For this review, take the finished solid that the model builds, in its own axes (mm). A direction names the side the tool comes from. Coordinates: 2 decimals unless noted, no trailing zeros. Loops run counter-clockwise (first coordinate to the right, second up) from the corner with the lowest first, then second, coordinate; pieces in that order, holes last. Notation, with made-up numbers: (22.25, 54.5) - (39.25, 54.5) arc R22 ccw to (39.25, 62.5) - close; hole circle Ø5 at (-12.5, 53). An arc over 180 degrees is marked (long way). Answer as a JSON object with one key per item and string values. Group by question number.
Item 1: Mouldability with a two-part tool opening along Y and no side actions: class faces 4 (the cylindrical face through (49.3, -26.87, -24.56)), 5 (the flat face through (49, 60.038, 11)), 6 (the flat face through (110, -4, 9)), 7 (the cylindrical face through (-4.93, -0.03, 8.67)) as released by +Y, released by -Y, zero draft, split by the parting line, or undercut.
Item 2: Clearance check with flat-ended pins moving along their axes: pin 1 (1.5 mm diameter, centred on x = 58.5, z = 0, fed in from -Y); pin 2 (6 mm diameter, centred on x = 28, y = -36, fed in from +Z); pin 3 (3 mm diameter, centred on x = 46.5, y = -30, fed in from +Z). State where each tip first meets the part, or that it passes through.
Item 3: To check wall thickness, follow line 1 (Z direction, x = 20, y = 50); line 2 (Y direction, x = 33, z = 0.5); line 3 (Y direction, x = 51.5, z = 13.5). State the ranges of each line that lie inside material, in increasing order.
Item 4: We need section D-D (y = -14.5). Give the boundary of the cut face in (x, z), then the cut area to 3 significant figures.
Item 5: We need section A-A (z = -22). Give the boundary of the cut face in (x, y), then the cut area to 3 significant figures.
Item 6: We need section C-C (z = -8). Give the boundary of the cut face in (x, y).
Item 7: Tool access review of faces 1 (the flat face through (-10, -4, 9)), 2 (the cylindrical face through (104.93, -0.03, 8.67)), 3 (the flat face through (49, -7.459, -6)): name each direction out of +Z, -Z, +X, -X, +Y, -Y from which nothing blocks a thin tool from reaching the whole face with its end or side.
from build123d import *

# Parameters (mm, degrees)
BOSS_EXTRU_1_DEPTH      = 100
ESQUISSE3_R             = 3.73
BOSS_EXTRU_2_DEPTH      = 10
BOSS_EXTRU_2_DEPTH_BACK = 110


with BuildPart() as part:
    # Esquisse1 → Boss.-Extru.1 (new body)
    with BuildSketch(Plane(origin=(0, 0, 0), x_dir=(0, 0, -1), z_dir=(1, 0, 0))):
        with BuildLine():
            Line((11.916237197, -42.931206961), (19.021149864, -50.036119628))
            ThreePointArc((19.021149864, -50.036119628), (35.155991103, -27.514297721), (38.400830806, 0))
            Line((38.400830806, 0), (38.400830806, 0.038210025))
            Line((38.400830806, 0.038210025), (-6.599169194, 0.038210025))
            Line((-6.599169194, 0.038210025), (-6.402631947, 60.038210025))
            Line((-6.402631947, 60.038210025), (-16.402685595, 60.038210025))
            Line((-16.402685595, 60.038210025), (-16.623781762, -7.459275773))
            Line((-16.623781762, -7.459275773), (28.904128187, -7.459275773))
            ThreePointArc((28.904128187, -7.459275773), (24.438110532, -27.124259516), (11.916237197, -42.931206961))
        make_face()
    extrude(amount=BOSS_EXTRU_1_DEPTH)

    # Esquisse3 → Boss.-Extru.2 (add, two sides)
    with BuildSketch(Plane.ZY) as boss_extru_2_sk:
        with Locations((9.151523675, -3.729275773)):
            Circle(ESQUISSE3_R)
    extrude(amount=BOSS_EXTRU_2_DEPTH)
    extrude(boss_extru_2_sk.sketch, amount=-BOSS_EXTRU_2_DEPTH_BACK)


solid = part.part
Check sheet entries:
{
 "1": {"face 4": "undercut", "face 5": "released by +Y", "face 6": "zero draft", "face 7": "split by the parting line"},
 "2": {"pin 1": "stops at y = -7.46", "pin 2": "stops at z = -16.21", "pin 3": "stops at z = -22.04"},
 "3": {"line 1": "z = 6.44 to 16.44", "line 2": "y = -7.46 to 0.04", "line 3": "y = -7.46 to 60.04"},
 "4": {"outline": "(0, -38.46) - (100, -38.46) - (100, -28.36) - (0, -28.36) - close", "area": "1,010 mm2"},
 "5": {"outline": "(0, -47.35) - (100, -47.35) - (100, -31.56) - (0, -31.56) - close; (0, -7.46) - (100, -7.46) - (100, 0.04) - (0, 0.04) - close", "area": "2,330 mm2"},
 "6": {"outline": "(0, -7.46) - (100, -7.46) - (100, 0.04) - (0, 0.04) - close"},
 "7": {"face 1": "+Z, -Z, -X, +Y, -Y", "face 2": "+X", "face 3": "+Z, +X, -X"}
}
